from build123d import *

# Parameters (mm, degrees)
SKETCH1_W           = 336.55
SKETCH1_H           = 88.9
BOSS_EXTRUDE1_DEPTH = 6.35
SKETCH2_W           = 30.48
SKETCH2_H           = 6.35
SKETCH2_W_2         = 6.35
SKETCH2_H_2         = 30.48
CUT_EXTRUDE1_DEPTH  = 7.35


with BuildPart() as part:
    # Sketch1 → Boss-Extrude1 (new body)
    with BuildSketch(Plane(origin=(0, 0, 0), x_dir=(1, 0, 0), z_dir=(0, 1, 0))):
        with Locations((-168.275, -44.45)):
            Rectangle(SKETCH1_W, SKETCH1_H)
    extrude(amount=BOSS_EXTRUDE1_DEPTH)

    # Sketch2 → Cut-Extrude1 (cut, through all)
    with BuildSketch(Plane(origin=(0, 6.35, 0), x_dir=(1, 0, 0), z_dir=(0, 1, 0))):
        with Locations((-168.275, -3.175)):
            Rectangle(SKETCH2_W, SKETCH2_H)
        with Locations((-168.275, -85.725)):
            Rectangle(SKETCH2_W, SKETCH2_H)
        with Locations((-3.175, -44.45)):
            Rectangle(SKETCH2_W_2, SKETCH2_H_2)
        with Locations((-333.375, -44.45)):
            Rectangle(SKETCH2_W_2, SKETCH2_H_2)
    extrude(amount=-CUT_EXTRUDE1_DEPTH, mode=Mode.SUBTRACT)


solid = part.part
Design review of the part built by this model. Coordinates are the model's own, in mm. A direction names the side the tool comes from. Give positions to 0.01 mm unless a question says otherwise; leave off trailing zeros. Loops run counter-clockwise (first coordinate to the right, second up) from the corner with the lowest first, then second, coordinate; pieces in that order, holes last. Notation, with made-up numbers: M -9,-32 L 18,-32 A29 cw 18,-12 Z; hole C 71,-17 d11. An arc over 180 degrees is marked long. Write item = value, one per line.
Q1. For faces 1 (the flat face through (-183.515, 3, 3)), 2 (the flat face through (-183.515, 3, 86)), 3 (the flat face through (-3, 3, 59.69)), 4 (the flat face through (-333, 3, 29.21)), list the 3-axis set-ups (+Z, -Z, +X, -X, +Y, -Y) from which the entire face can be reached by the end or side of a thin tool; tool diameter is ignored.
Output values:
face_1 = -Z, +Y, -Y
face_2 = +Z, +Y, -Y
face_3 = +X, +Y, -Y
face_4 = -X, +Y, -Y
Q2. We need section B-B (z = 47). Give the boundary of the cut face in (x, y).
Output values:
outline = M -330.2,0 L -6.35,0 L -6.35,6.35 L -330.2,6.35 Z
Q3. To check wall thickness, follow line 1 (X direction, y = 3.75, z = 42). State the ranges of the line that lie inside material, in increasing order. Write a range as [from, to].
Output values:
line_1 = [-330.2, -6.35]
Q4. Draft analysis for pull direction X (two halves, no side actions). For faces 5 (the flat face through (-168, 3, 6.35)), 6 (the flat face through (-6.35, 3, 45)), 7 (the flat face through (-153.035, 3, 86)), 8 (the flat face through (-261, 3, 0)), state which applies: +X half, -X half, draft (parallel to the pull), parting line (faces both ways), or undercut.
Output values:
face_5 = undercut
face_6 = +X half
face_7 = undercut
face_8 = draft
Q5. We need section A-A (y = 1.75). Give the boundary of the cut face in (x, z) (3 decimals), plus the area to 3 significant figures.
Output values:
outline = M -336.55,0 L -183.515,0 L -183.515,6.35 L -153.035,6.35 L -153.035,0 L 0,0 L 0,29.21 L -6.35,29.21 L -6.35,59.69 L 0,59.69 L 0,88.9 L -153.035,88.9 L -153.035,82.55 L -183.515,82.55 L -183.515,88.9 L -336.55,88.9 L -336.55,59.69 L -330.2,59.69 L -330.2,29.21 L -336.55,29.21 Z
area = 29,100 mm^2
Q6. Insertion check: pin 1 (1.9 mm diameter, centred on x = -171, y = 4, fed in from +Z). The pin has a flat end and moves straight along its axis. Give the tip position at first contact, or say it passes through.
Output values:
pin_1 = 82.55
